```python
from build123d import *

# Parameters (mm, degrees)
EXTRUDE_2_DEPTH = 4


with BuildPart() as part:
    # Sketch 1 → Бобышка-Вытянуть2 (new body)
    with BuildSketch(Plane(origin=(9.520291442, 10, -132.987365348), x_dir=(0, 0, 1), z_dir=(0, -1, 0))):
        Polygon((0, 0), (300, 0), (184.59311112, 175.445860593), (84.59311112, 175.445860593), align=None)
        Polygon((83.826194839, 143.144403483), (83.826194839, 36.144403483), (175.826194839, 36.144403483), (175.826194839, 143.144403483), (147.826194839, 170.445860593), (111.826194839, 170.445860593), align=None, mode=Mode.SUBTRACT)
    extrude(amount=-EXTRUDE_2_DEPTH)


solid = part.part
```
Read the model definition and answer for the solid it produces. Units are mm, in the model's axes. A direction names the side the tool comes from. Coordinates: 2 decimals unless noted, no trailing zeros. Write each loop counter-clockwise with the first axis right and the second up, starting at its lowest first coordinate (ties: lowest second). Pieces come first, ordered by that corner, then holes. Notation, with made-up numbers: (-21.75, 69.25) -> (34.25, 69.25) arc R38 cw to (34.25, 108.25) -> close; hole circle Ø6 at (-21, -31.75). An arc over 180 degrees is marked (long way). Answer as a JSON object with one key per item and string values.
Q1. The part is cut by section D-D on z = -61. Give the vertices of the cut face in (x, y).
The answers:
{"outline": "(-139.78, 10) -> (9.52, 10) -> (9.52, 14) -> (-139.78, 14) -> close"}
Q2. Flat-ended cylindrical pins translate along their axes: pin 1 Ø2 at (x, y) = (-59.5, 12.5) entering from -Z; pin 2 Ø1 at (x, y) = (-98.5, 11.5) entering from +Z. Find the tip coordinate at first contact, or state that the pin passes through.
The answers:
{"pin 1": "stops at z = -100.19", "pin 2": "stops at z = 96.29"}
Q3. A tool of negligible diameter and unlimited length cuts with its end or side. For faces 1 (the flat face through (-79.43, 11.97, -90.1)), 2 (the flat face through (-147.084, 11.972, 29.035)), from which of +Z, -Z, +X, -X, +Y, -Y can it reach the whole face along a straight path? Write none if from no direction.
The answers:
{"face 1": "-Z, -X, +Y, -Y", "face 2": "+Y, -Y"}
Q4. Consider line 1 (X direction, y = 11.6, z = 0.5); line 2 (Z direction, x = -63, y = 13.8); line 3 (Z direction, x = -86, y = 12.4). Determine where each line is inside the solid, lowest interval first. Write a range as [from, to].
The answers:
{"line 1": "x = [-165.93, -160.93], [-26.62, 9.52]", "line 2": "z = [-98.02, -49.16], [42.84, 119.31]", "line 3": "z = [-86.93, -49.16], [42.84, 104.18]"}
Q5. The part is cut by section C-C on x = -55. Give the vertices of the cut face in (y, z).
The answers:
{"outline": "(10, -101.88) -> (14, -101.88) -> (14, -49.16) -> (10, -49.16) -> close; (10, 42.84) -> (14, 42.84) -> (14, 124.57) -> (10, 124.57) -> close"}
Q6. The part is cut by section A-A on z = 9. Give the vertices of the cut face in (x, y), then the cut area to 3 significant figures.
The answers:
{"outline": "(-165.93, 10) -> (-160.93, 10) -> (-160.93, 14) -> (-165.93, 14) -> close; (-26.62, 10) -> (9.52, 10) -> (9.52, 14) -> (-26.62, 14) -> close", "area": "165 mm2"}
Q7. Determine the mould class of faces 3 (the flat face through (-60, 10, 48)), 4 (the flat face through (-77, 12, 110.1)), 5 (the flat face through (-147.466, 11.972, -34.965)) for opening direction Z: pulls with the +Z half, pulls with the -Z half, needs draft (parallel to the pull), parting line crosses it, or undercut.
The answers:
{"face 3": "needs draft", "face 4": "pulls with the +Z half", "face 5": "undercut"}
Q8. The part is cut by section B-B on y = 12.15. Give the vertices of the cut face in (x, z), then the cut area to 3 significant figures.
The answers:
{"outline": "(-165.93, -48.39) -> (9.52, -132.99) -> (9.52, 167.01) -> (-165.93, 51.61) -> close; hole (-160.93, -21.16) -> (-133.62, -49.16) -> (-26.62, -49.16) -> (-26.62, 42.84) -> (-133.62, 42.84) -> (-160.93, 14.84) -> close", "area": "23,500 mm2"}
